```python
from build123d import *

# Parameters (mm, degrees)
SKETCH1_W               = 254
SKETCH1_H               = 70
BOSS_EXTRUDE1_DEPTH     = 3.175
F_8_32_TAPPED_HOLE1_D   = 4.1656
F_6_32_TAPPED_HOLE1_D   = 3.5052
F_1_4_20_TAPPED_HOLE1_D = 6.35
F_8_32_TAPPED_HOLE2_D   = 4.1656


with BuildPart() as part:
    # Sketch1 → Boss-Extrude1 (new body)
    with BuildSketch(Plane.XY):
        with Locations((127, 35)):
            Rectangle(SKETCH1_W, SKETCH1_H)
    extrude(amount=BOSS_EXTRUDE1_DEPTH)

    # #8-32 Tapped Hole1 (through all)
    with Locations(Plane.XY.offset(3.175)):
        with Locations((228.6, 62.187398), (196.85, 35), (95.25, 35), (120.65, 35), (146.05, 35), (133.35, 35), (107.95, 35)):
            Hole(F_8_32_TAPPED_HOLE1_D / 2)

    # #6-32 Tapped Hole1 (through all)
    with Locations(Plane.XY.offset(3.175)):
        with Locations((36.673632472, 66.368109228), (83.972588612, 66.324919192), (83.972588612, 3.675080808), (36.673632472, 3.631890772)):
            Hole(F_6_32_TAPPED_HOLE1_D / 2)

    # 1/4-20 Tapped Hole1 (through all)
    with Locations(Plane.XY.offset(3.175)):
        with Locations((12.7, 57.3), (241.3, 12.7), (241.3, 57.3), (12.7, 12.7)):
            Hole(F_1_4_20_TAPPED_HOLE1_D / 2)

    # #8-32 Tapped Hole2 (through all)
    with Locations(Plane.XY.offset(3.175)):
        with Locations((228.6, 35.199898), (196.85, 8.0125), (120.65, 8.0125)):
            Hole(F_8_32_TAPPED_HOLE2_D / 2)


solid = part.part
```
For this review, take the finished solid that the model builds, in its own axes (mm). Give positions to 0.01 mm unless a question says otherwise; leave off trailing zeros. Write each loop counter-clockwise with the first axis right and the second up, starting at its lowest first coordinate (ties: lowest second). Pieces come first, ordered by that corner, then holes. Notation, with made-up numbers: M 78.5,37.5 L 92.5,37.5 A18 cw 92.5,63.5 Z; hole C 44.5,18 d1. An arc over 180 degrees is marked long. Answer as a JSON object with one key per item and string values. Group by question number.
Item 1: Consider section B-B on x = 12.7. Write out the cut boundary in (y, z) (3 decimals), plus the area to 3 significant figures.
Item 2: Consider section C-C on z = 1.3. Count the separate pieces of the cut face and the enclosed holes in it, plus the area to 3 significant figures.
Item 3: For probe 1 along Y at (x, z) = (196.85, 0.7); probe 2 along X at (y, z) = (57.5, 2.2); probe 3 along Y at (x, z) = (228.6, 2.5), list the stretches that pass through material, from the lowest coordinate up. Write a range as [from, to].
Item 4: Consider section A-A on y = 57.3. Write out the cut boundary in (x, z) (3 decimals).
Item 5: For pin 1 Ø6.5 at (x, y) = (107.95, 35) entering from +Z (3 decimals), flat-tipped, find the tip position at first contact; note if it passes through.
Item 6: Draft analysis for pull direction X (two halves, no side actions). For faces 1 (the flat face through (125, 35, 0)), 2 (the cylindrical face through (13.11, 60.45, 1.57)), state which applies: +X half, -X half, draft (parallel to the pull), parting line (faces both ways), or undercut.
Check result:
{
 "1": {"outline": "M 0,0 L 9.525,0 L 9.525,3.175 L 0,3.175 Z; M 15.875,0 L 54.125,0 L 54.125,3.175 L 15.875,3.175 Z; M 60.475,0 L 70,0 L 70,3.175 L 60.475,3.175 Z", "area": "182 mm^2"},
 "2": {"separate pieces": "1", "enclosed holes": "18", "area": "17,500 mm^2"},
 "3": {"probe 1": "y = [0, 5.93], [10.1, 32.92], [37.08, 70]", "probe 2": "x = [0, 9.53], [15.87, 238.13], [244.47, 254]", "probe 3": "y = [0, 33.12], [37.28, 60.1], [64.27, 70]"},
 "4": {"outline": "M 0,0 L 9.525,0 L 9.525,3.175 L 0,3.175 Z; M 15.875,0 L 238.125,0 L 238.125,3.175 L 15.875,3.175 Z; M 244.475,0 L 254,0 L 254,3.175 L 244.475,3.175 Z"},
 "5": {"pin 1": "stops at z = 3.175"},
 "6": {"face 1": "draft", "face 2": "undercut"}
}
